CAD build for the part. Positions are in the model's coordinates, mm. A direction names the side the tool comes from. Give positions to 0.01 mm unless a question says otherwise; leave off trailing zeros. Write each loop counter-clockwise with the first axis right and the second up, starting at its lowest first coordinate (ties: lowest second). Pieces come first, ordered by that corner, then holes. Notation, with made-up numbers: (21.25, -40) -> (26.25, -40) arc R18 cw to (26.25, -18) -> close; hole circle Ø3 at (63, 23). An arc over 180 degrees is marked (long way). Answer as a JSON object with one key per item and string values.
```python
from build123d import *

# Parameters (mm, degrees)
CUT_EXTRUDE1_START  = 3
CUT_EXTRUDE1_DEPTH  = 10
FILLET1_R           = 1
CHAMFER1_SIZE       = 0.5
CHAMFER2_SIZE       = 0.5
SKETCH3_R           = 4.1
BOSS_EXTRUDE1_DEPTH = 15


# Read off the part's stored shape, not the designer's step: M8x1.0 Machine Threads Stud1
with BuildPart() as part:
    # Sketch1 → Revolve1 (revolve)
    with BuildSketch(Plane(origin=(0, 0, 0), x_dir=(1, 0, 0), z_dir=(0, 1, 0))):
        Polygon((0, 0), (0, -5), (93, -5), (93, -7.5), (123, -7.5), (123, -9), (169, -9), (169, -5), (184, -5), (184, 0), align=None)
    revolve(axis=Axis((0, 0, 0), (1, 0, 0)))

    # Sketch2 → Cut-Extrude1 (cut)
    with BuildSketch(Plane(origin=(0, 0, 0), x_dir=(1, 0, 0), z_dir=(0, 1, 0)).offset(CUT_EXTRUDE1_START)):
        with BuildLine():
            Line((-11, -1.5), (11, -1.5))
            ThreePointArc((11, -1.5), (12.5, 0), (11, 1.5))
            Line((11, 1.5), (-11, 1.5))
            Line((-11, 1.5), (-11, -1.5))
        make_face()
    extrude(amount=CUT_EXTRUDE1_DEPTH, mode=Mode.SUBTRACT)

    # Fillet1
    fillet1_edges = [part.edges().sort_by_distance(p)[0] for p in [
        (123, 0, -7.5),
        (93, 0, -5),
        (169, 0, -5),
    ]]
    fillet(fillet1_edges, radius=FILLET1_R)

    # Chamfer1
    chamfer1_edges = [part.edges().sort_by_distance(p)[0] for p in [
        (0, -4.031128874, -2.958039892),
    ]]
    chamfer(chamfer1_edges, length=CHAMFER1_SIZE)

    # Chamfer2
    chamfer2_edges = [part.edges().sort_by_distance(p)[0] for p in [
        (184, 0, -5),
        (169, 0, -9),
    ]]
    chamfer(chamfer2_edges, length=CHAMFER2_SIZE)

    # Sketch3 → Boss-Extrude1 (add)
    with BuildSketch(Plane(origin=(184, 0, 0), x_dir=(0, 0, -1), z_dir=(1, 0, 0))):
        Circle(SKETCH3_R)
    extrude(amount=BOSS_EXTRUDE1_DEPTH)

    # M8x1.0 Machine Threads Stud1 outline → M8x1.0 Machine Threads Stud1 (revolve, cut)
    with BuildSketch(Plane.YX):
        with BuildLine():
            ThreePointArc((3, 184.4), (3.117157288, 184.117157288), (3.4, 184))
            Line((3.4, 184), (4.1, 184))
            Line((4.1, 184), (4.1, 199))
            Line((4.1, 199), (3.4455, 199))
            Line((3.4455, 199), (4, 198.4455))
            Line((4, 198.4455), (4, 186.939230485))
            Line((4, 186.939230485), (3.053589838, 185.3))
            ThreePointArc((3.053589838, 185.3), (3.013629669, 185.203527618), (3, 185.1))
            Line((3, 185.1), (3, 184.4))
        make_face()
    revolve(axis=Axis((0, 0, 0), (1, 0, 0)), mode=Mode.SUBTRACT)


solid = part.part
```
1) Slice it at B-B (x = 149.5). List the corners of the cut face in (y, z).
Model answer:
{"outline": "circle Ø18 at (0, 0)"}
2) Pin check, flat tips, straight feed: pin 1 (2 mm diameter, centred on x = 59, y = 5.5, fed in from +Z); pin 2 (2 mm diameter, centred on y = 7, z = 0, fed in from -X); pin 3 (1 mm diameter, centred on x = 65, y = 0, fed in from +Z). Stop position of each tip, or through.
Model answer:
{"pin 1": "stops at z = 2.18", "pin 2": "stops at x = 93", "pin 3": "stops at z = 5"}
3) Slice it at A-A (x = 64). List the corners of the cut face in (y, z).
Model answer:
{"outline": "circle Ø10 at (0, 0)"}
4) Mould opens along X. For faces 4 (the conical face through (0.135, -4.632, 0.184)), 5 (the flat face through (169, -6, 2)), 6 (the cylindrical face through (176.84, 4.88, -1.08)), 7 (the cylindrical face through (184.7, -3, 0.1)) say: released by +X, released by -X, zero draft, split by the parting line, or undercut.
Model answer:
{"face 4": "released by -X", "face 5": "released by +X", "face 6": "zero draft", "face 7": "undercut"}
5) Wall check: probe 1 along X at (y, z) = (2.25, 6.5); probe 2 along Y at (x, z) = (25, 4); probe 3 along X at (y, z) = (-0.5, -4.5). Give the ranges that are in metal, low to high.
Model answer:
{"probe 1": "x = 93 to 169", "probe 2": "y = -3 to 3", "probe 3": "x = 0.03 to 183.97"}
6) 3-axis set-ups, long thin cutter, end or side, ignore diameter. For faces 1 (the cylindrical face through (107.703, -0.33, -7.493)), 2 (the cylindrical face through (192.612, -0.867, -3.905)), 3 (the flat face through (184, -3, -2)): which of +Z, -Z, +X, -X, +Y, -Y reach the whole face in a straight line?
Model answer:
{"face 1": "-X", "face 2": "+X", "face 3": "none"}
